from build123d import *

# Parameters (mm, degrees)
SKETCH2_R           = 30
BOSS_EXTRUDE1_DEPTH = 5
SKETCH3_W           = 40
SKETCH3_H           = 20
CUT_EXTRUDE1_DEPTH  = 6
SKETCH4_W           = 20
SKETCH4_H           = 5
CUT_EXTRUDE2_DEPTH  = 10
SKETCH5_R           = 2.1
CUT_EXTRUDE3_DEPTH  = 6


with BuildPart() as part:
    # Sketch2 → Boss-Extrude1 (new body)
    with BuildSketch(Plane(origin=(0, 0, 0), x_dir=(1, 0, 0), z_dir=(0, 1, 0))):
        Circle(SKETCH2_R)
    extrude(amount=BOSS_EXTRUDE1_DEPTH)

    # Sketch3 → Cut-Extrude1 (cut, through all)
    with BuildSketch(Plane(origin=(0, 5, 0), x_dir=(1, 0, 0), z_dir=(0, 1, 0))):
        Rectangle(SKETCH3_W, SKETCH3_H)
    extrude(amount=-CUT_EXTRUDE1_DEPTH, mode=Mode.SUBTRACT)

    # Sketch4 → Cut-Extrude2 (cut)
    with BuildSketch(Plane(origin=(0, 5, 0), x_dir=(1, 0, 0), z_dir=(0, 1, 0))):
        with Locations((-5, 17.5)):
            Rectangle(SKETCH4_W, SKETCH4_H)
        with Locations((-5, -17.5)):
            Rectangle(SKETCH4_W, SKETCH4_H)
    extrude(amount=-CUT_EXTRUDE2_DEPTH, mode=Mode.SUBTRACT)

    # Sketch5 → Cut-Extrude3 (cut, through all)
    with BuildSketch(Plane.XZ):
        with Locations((-24.761145618, -5.075)):
            Circle(SKETCH5_R)
        with Locations((-24.761145618, 4.775)):
            Circle(SKETCH5_R)
        with Locations((24.661145618, 4.775)):
            Circle(SKETCH5_R)
        with Locations((24.661145618, -5.075)):
            Circle(SKETCH5_R)
    extrude(amount=-CUT_EXTRUDE3_DEPTH, mode=Mode.SUBTRACT)


solid = part.part
Input: part model. Units: mm. Frame: model coordinates. Coordinates: 2 decimals unless noted, no trailing zeros. Order: outer loops, then holes, each group sorted by start corner. A loop starts at its lowest first (then second) coordinate and runs counter-clockwise, first axis right, second up. Notation, with made-up numbers: M 39,29 L 49,29 A18 cw 49,47 Z; hole C 37,-31 d9. An arc over 180 degrees is marked long. Answer in a Markdown table with one row per item.
(1) Section query B-B, the plane x = 0. Output: boundary loops of the cut face in (y, z).
Numbers:
| item | result |
|---|---|
| outline | M 0,-30 L 5,-30 L 5,-20 L 0,-20 Z; M 0,-15 L 5,-15 L 5,-10 L 0,-10 Z; M 0,10 L 5,10 L 5,15 L 0,15 Z; M 0,20 L 5,20 L 5,30 L 0,30 Z |
(2) Section query D-D, the plane y = 3.6. Output: boundary loops of the cut face in (x, z) (3 decimals).
Numbers:
| item | result |
|---|---|
| outline | C 0,0 d60; hole C -24.761,-5.075 d4.2; hole C -24.761,4.775 d4.2; hole M -20,-10 L 20,-10 L 20,10 L -20,10 Z; hole M -15,-20 L 5,-20 L 5,-15 L -15,-15 Z; hole M -15,15 L 5,15 L 5,20 L -15,20 Z; hole C 24.661,-5.075 d4.2; hole C 24.661,4.775 d4.2 |
(3) Contact query for flat-ended pins moving along their axis: pin 1 Ø1 at (y, z) = (2, -13) entering from -X; pin 2 Ø1.5 at (y, z) = (1.5, -18.5) entering from +X; pin 3 Ø2.5 at (y, z) = (3.5, -18.5) entering from -X. Output: stop coordinate, or through.
Numbers:
| item | result |
|---|---|
| pin 1 | stops at x = -27.27 |
| pin 2 | stops at x = 24.19 |
| pin 3 | stops at x = -24.54 |
(4) Draft query along Z for faces 1 (the flat face through (-15, 3, -17)), 2 (the flat face through (0, 0, -14)), 3 (the cylindrical face through (-29.97, 2.46, -1.32)). Return one class per face: pulls with the +Z half, pulls with the -Z half, needs draft (parallel to the pull), parting line crosses it, or undercut.
Numbers:
| item | result |
|---|---|
| face 1 | undercut |
| face 2 | needs draft |
| face 3 | parting line crosses it |
(5) Section query A-A, the plane z = 0. Output: boundary loops of the cut face in (x, y), plus the area to 3 significant figures.
Numbers:
| item | result |
|---|---|
| outline | M -30,0 L -20,0 L -20,5 L -30,5 Z; M 20,0 L 30,0 L 30,5 L 20,5 Z |
| area | 100 mm^2 |
(6) Material intervals for line 1 (Z direction, x = 0.5, y = 4.4); line 2 (Z direction, x = -6, y = 0.75); line 3 (Z direction, x = 25, y = 4.5), sorted ascending. Write a range as [from, to].
Numbers:
| item | result |
|---|---|
| line 1 | z = [-30, -20], [-15, -10], [10, 15], [20, 30] |
| line 2 | z = [-29.39, -20], [-15, -10], [10, 15], [20, 29.39] |
| line 3 | z = [-16.58, -7.15], [-3, 2.7], [6.85, 16.58] |
(7) Section query C-C, the plane x = 10.5. Output: boundary loops of the cut face in (y, z), plus the area to 3 significant figures.
Numbers:
| item | result |
|---|---|
| outline | M 0,-28.1 L 5,-28.1 L 5,-10 L 0,-10 Z; M 0,10 L 5,10 L 5,28.1 L 0,28.1 Z |
| area | 181 mm^2 |
